Design review of the part built by this model. Coordinates are the model's own, in mm. Face numbers are marked on the shaded views. Coordinates: 2 decimals unless noted, no trailing zeros. Loops run counter-clockwise (first coordinate to the right, second up) from the corner with the lowest first, then second, coordinate; pieces in that order, holes last. Notation, with made-up numbers: (10, 67) -> (52, 67) arc R5 ccw to (52, 72) -> close; hole circle Ø2 at (72, -14). An arc over 180 degrees is marked (long way). Use a Markdown table: item, result. Add a question column.
Q1. Take a section at D-D on x = -19. Write out the cut boundary in (y, z).
Q2. Clearance check with flat-ended pins moving along their axes: pin 1 Ø11 at (x, y) = (19.2, 0) entering from +Z; pin 2 Ø1 at (x, z) = (-17.5, 0.5) entering from +Y. State where each tip first meets the part, or that it passes through.
Q3. For probe 1 along Y at (x, z) = (0, 1.45); probe 2 along X at (y, z) = (-12, 2.05); probe 3 along Y at (x, z) = (19.5, 2.6), list the stretches that pass through material, from the lowest coordinate up.
Q4. Take a section at C-C on z = 2.25. Write out the cut boundary in (x, y).
Q5. Draft analysis for pull direction X (two halves, no side actions). For the marked faces 1, 2 and 3, state which applies: pulls with the +X half, pulls with the -X half, needs draft (parallel to the pull), parting line crosses it, or undercut.
Q6. Take a section at A-A on x = 0. Write out the cut boundary in (y, z), plus the area to 3 significant figures.
from build123d import *

# Parameters (mm, degrees)
CYLINDER_R     = 26.7
CYLINDER_DEPTH = 3
SKETCH_R       = 3.5
POCKET_DEPTH   = 3


with BuildPart() as part:
    # Cylinder → Cylinder (new body)
    with BuildSketch(Plane.XY):
        Circle(CYLINDER_R)
    extrude(amount=CYLINDER_DEPTH)

    # Sketch → Pocket (cut)
    with BuildSketch(Plane.XY.offset(3)):
        with Locations((0, 19.2)):
            Circle(SKETCH_R)
        with Locations((16.6277, -9.6)):
            Circle(SKETCH_R)
        with Locations((-16.6277, -9.6)):
            Circle(SKETCH_R)
        with Locations((0, -19.2)):
            Circle(SKETCH_R)
        with Locations((-19.2, 0)):
            Circle(SKETCH_R)
        with Locations((19.2, 0)):
            Circle(SKETCH_R)
        with BuildLine():
            ThreePointArc((7.688102, 8.819472), (-8.273149, -8.273149), (8.819472, 7.688102))
            Line((8.819472, 7.688102), (9.333811, 8.202441))
            ThreePointArc((9.333811, 8.202441), (9.899497, 9.899497), (8.202441, 9.333811))
            Line((7.688102, 8.819472), (8.202441, 9.333811))
        make_face()
    extrude(amount=-POCKET_DEPTH, mode=Mode.SUBTRACT)


solid = part.part
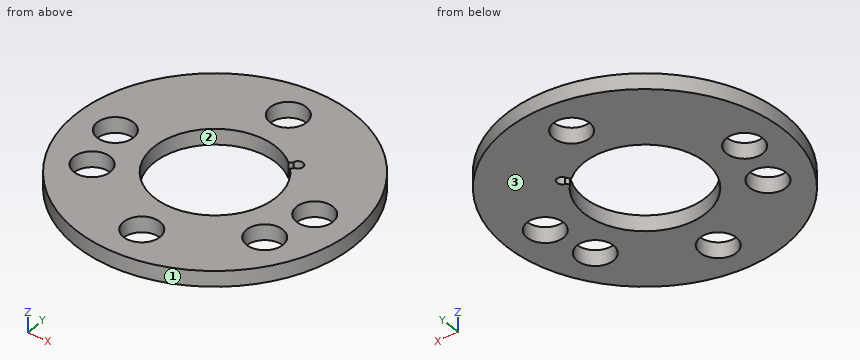
Answer list:
| question | item | result |
|---|---|---|
| 1 | outline | (-18.76, 0) -> (-12.17, 0) -> (-12.17, 3) -> (-18.76, 3) -> close; (-7.03, 0) -> (-3.49, 0) -> (-3.49, 3) -> (-7.03, 3) -> close; (3.49, 0) -> (18.76, 0) -> (18.76, 3) -> (3.49, 3) -> close |
| 2 | pin 1 | z = 3 |
| 2 | pin 2 | y = 20.59 |
| 3 | probe 1 | -26.7 to -22.7, -15.7 to -11.7, 11.7 to 15.7, 22.7 to 26.7 |
| 3 | probe 2 | -23.85 to -19.18, -14.08 to 14.08, 19.18 to 23.85 |
| 3 | probe 3 | -18.24 to -11.6, -7.6 to -3.49, 3.49 to 18.24 |
| 4 | outline | circle Ø53.4 at (0, 0); hole circle Ø7 at (-19.2, 0); hole circle Ø7 at (-16.63, -9.6); hole circle Ø7 at (0, -19.2); hole circle Ø7 at (0, 19.2); hole (7.69, 8.82) arc R11.7 ccw (long way) to (8.82, 7.69) -> (9.33, 8.2) arc R1 ccw (long way) to (8.2, 9.33) -> close; hole circle Ø7 at (16.63, -9.6); hole circle Ø7 at (19.2, 0) |
| 5 | face 1 | parting line crosses it |
| 5 | face 2 | undercut |
| 5 | face 3 | needs draft |
| 6 | outline | (-26.7, 0) -> (-22.7, 0) -> (-22.7, 3) -> (-26.7, 3) -> close; (-15.7, 0) -> (-11.7, 0) -> (-11.7, 3) -> (-15.7, 3) -> close; (11.7, 0) -> (15.7, 0) -> (15.7, 3) -> (11.7, 3) -> close; (22.7, 0) -> (26.7, 0) -> (26.7, 3) -> (22.7, 3) -> close |
| 6 | area | 48.0 mm² |
